Part model, mm, in its own coordinate system. Face numbers are marked on the shaded views. A direction names the side the tool comes from. Give positions to 0.01 mm unless a question says otherwise; leave off trailing zeros. Order: outer loops, then holes, each group sorted by start corner. A loop starts at its lowest first (then second) coordinate and runs counter-clockwise, first axis right, second up. Notation, with made-up numbers: (26.5, 45) -> (54.5, 45) arc R7 cw to (54.5, 51) -> close; hole circle Ø6 at (39, 77.25). An arc over 180 degrees is marked (long way). Write item = value, one per line. Start each with the question number.
Item 1: Flat gauge pins, fed straight in: P1, Ø3, axis at y = 25.5, z = -1, coming from the -X side; P2, Ø2, axis at y = -9.5, z = -5, coming from the -X side; P3, Ø7, axis at y = -23, z = -2.5, coming from the -X side; P4, Ø5, axis at y = -6, z = 5, coming from the -X side. Where does each tip first touch, or does it go through?
Item 2: Band-saw the part on B-B on x = 0. Write the cut outline in (y, z).
Item 3: Pull direction Z, two halves, no side cores. Call the marked faces 1, 2, 3 and 4: +Z half, -Z half, draft (parallel to the pull), parting line (faces both ways), or undercut.
Item 4: Drill centre lines: line 1 along Y through (x, z) = (0, 12.7); line 2 along Y through (x, z) = (0.5, 11.25); line 3 along X through (y, z) = (19, 10.5). Where is each one in solid material? Low to high.
Item 5: Band-saw the part on C-C on z = 3.5. Write the cut outline in (x, y), plus the area to 3 significant figures.
Item 6: Tool access for the marked faces 5, 6 and 7: list every direction of +Z, -Z, +X, -X, +Y, -Y with a clear straight run to the whole face (end or side of a thin tool).
Item 7: Band-saw the part on A-A on y = 0. Write the cut outline in (x, z), plus the area to 3 significant figures.
Item 8: Band-saw the part on D-D on y = -10. Write the cut outline in (x, z).
```python
from build123d import *

# Parameters (mm, degrees)
F3_W      = 25.4
F3_H      = 12.7
F4_DEPTH  = 72.39
F7_DEPTH  = 53.086
F10_DEPTH = 47.244


# Not quite as in the source:
# - a feature names something its author has since deleted; it is built from what else it names


with BuildPart() as f1:
    # F0 (on Front) → F1 (revolve)
    with BuildSketch(Plane.XZ):
        with BuildLine():
            ThreePointArc((23.01875, 10.7376509739), (25.4, 0), (23.01875, -10.7376509739))
            Line((23.01875, -10.7376509739), (23.01875, -14.2875))
            Line((23.01875, -14.2875), (26.611533725, -14.2875))
            ThreePointArc((26.611533725, -14.2875), (30.20441, 0), (26.611533725, 14.2875))
            Line((26.611533725, 14.2875), (23.01875, 14.2875))
            Line((23.01875, 14.2875), (23.01875, 10.7376509739))
        make_face()
    revolve(axis=Axis((0, 0, -4.5421977431), (0, 0, -1)))

    # F3 (on offset) → F4 (cut)
    with BuildSketch(Plane.XZ.offset(30.20441)):
        with BuildLine():
            ThreePointArc((12.7, 6.35), (0, 9.7529547439), (-12.7, 6.35))
            Line((-12.7, 6.35), (12.7, 6.35))
        make_face()
        Rectangle(F3_W, F3_H)
        with BuildLine():
            Line((12.7, -6.35), (-12.7, -6.35))
            ThreePointArc((-12.7, -6.35), (0, -9.7529547439), (12.7, -6.35))
        make_face()
    extrude(amount=-F4_DEPTH, mode=Mode.SUBTRACT)

    # F6 (on line) → F7 (cut, symmetric)
    with BuildSketch(Plane(origin=(0, 0, 0), x_dir=(0.5, -0.8660254038, 0), z_dir=(-0.8660254038, -0.5, 0))):
        with BuildLine():
            ThreePointArc((6.6390036837, -7.9375), (10.34796, 0), (6.6390036837, 7.9375))
            Line((6.6390036837, 7.9375), (-6.6390036837, 7.9375))
            ThreePointArc((-6.6390036837, 7.9375), (-10.34796, 0), (-6.6390036837, -7.9375))
            Line((-6.6390036837, -7.9375), (6.6390036837, -7.9375))
        make_face()
    extrude(amount=F7_DEPTH, both=True, mode=Mode.SUBTRACT)

    # F9 (on line) → F10 (cut, symmetric)
    with BuildSketch(Plane(origin=(0, 0, 0), x_dir=(-0.5, -0.8660254038, 0), z_dir=(-0.8660254038, 0.5, 0))):
        with BuildLine():
            ThreePointArc((6.6390036837, -7.9375), (10.34796, 0), (6.6390036837, 7.9375))
            Line((6.6390036837, 7.9375), (-6.6390036837, 7.9375))
            ThreePointArc((-6.6390036837, 7.9375), (-10.34796, 0), (-6.6390036837, -7.9375))
            Line((-6.6390036837, -7.9375), (6.6390036837, -7.9375))
        make_face()
    extrude(amount=F10_DEPTH, both=True, mode=Mode.SUBTRACT)


solid = f1.part
```
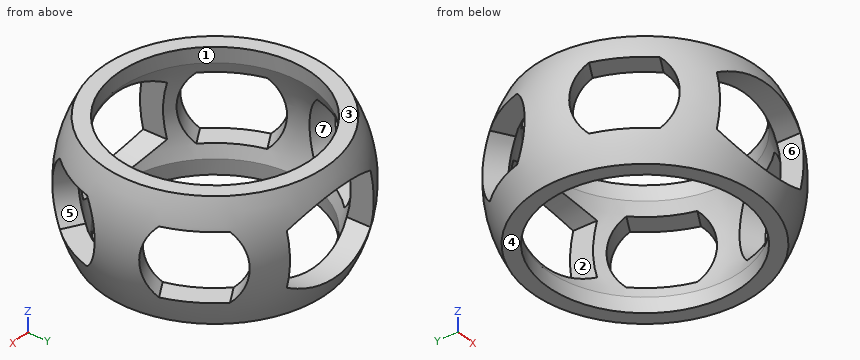
Values found:
q1.P1 = -18.31
q1.P2 = through
q1.P3 = -20.27
q1.P4 = -29.73
q2.outline = (-28.59, -9.75) arc R30.2 ccw to (-26.61, -14.29) -> (-23.02, -14.29) -> (-23.02, -10.74) arc R25.4 cw to (-23.45, -9.75) -> close; (-28.59, 9.75) -> (-23.45, 9.75) arc R25.4 cw to (-23.02, 10.74) -> (-23.02, 14.29) -> (-26.61, 14.29) arc R30.2 ccw to start; (23.02, -14.29) -> (26.61, -14.29) arc R30.2 ccw to (28.59, -9.75) -> (23.45, -9.75) arc R25.4 cw to (23.02, -10.74) -> close; (23.02, 10.74) arc R25.4 cw to (23.45, 9.75) -> (28.59, 9.75) arc R30.2 ccw to (26.61, 14.29) -> (23.02, 14.29) -> close
q3.face_1 = draft
q3.face_2 = undercut
q3.face_3 = +Z half
q3.face_4 = -Z half
q4.line_1 = -27.4 to -23.02, 23.02 to 27.4
q4.line_2 = -28.03 to -23.01, 23.01 to 28.03
q4.line_3 = -21 to -13.19, 13.19 to 21
q5.outline = (-29.44, -5.75) -> (-24.96, -3.16) arc R25.16 cw to (-24.96, 3.16) -> (-29.44, 5.75) arc R30 ccw to start; (-19.71, -22.62) arc R30 ccw to (-12.7, -27.18) -> (-12.7, -21.72) arc R25.16 cw to (-15.22, -20.03) -> close; (-19.71, 22.62) -> (-15.22, 20.03) arc R25.16 cw to (-12.7, 21.72) -> (-12.7, 27.18) arc R30 ccw to start; (12.7, -27.18) arc R30 ccw to (19.71, -22.62) -> (15.22, -20.03) arc R25.16 cw to (12.7, -21.72) -> close; (12.7, 21.72) arc R25.16 cw to (15.22, 20.03) -> (19.71, 22.62) arc R30 ccw to (12.7, 27.18) -> close; (24.96, -3.16) -> (29.44, -5.75) arc R30 ccw to (29.44, 5.75) -> (24.96, 3.16) arc R25.16 cw to start
q5.area = 198 mm^2
q6.face_5 = +X
q6.face_6 = +Y, -Y
q6.face_7 = +Y
q7.outline = (-26.61, -14.29) -> (-23.02, -14.29) -> (-23.02, -10.74) arc R25.4 cw to (-23.02, 10.74) -> (-23.02, 14.29) -> (-26.61, 14.29) arc R30.2 ccw to start; (23.02, -14.29) -> (26.61, -14.29) arc R30.2 ccw to (26.61, 14.29) -> (23.02, 14.29) -> (23.02, 10.74) arc R25.4 cw to (23.02, -10.74) -> close
q7.area = 275 mm^2
q8.outline = (-27.37, -7.94) arc R28.5 ccw to (-24.66, -14.29) -> (-20.73, -14.29) -> (-20.73, -10.74) arc R23.35 cw to (-21.96, -7.94) -> close; (-27.37, 7.94) -> (-21.96, 7.94) arc R23.35 cw to (-20.73, 10.74) -> (-20.73, 14.29) -> (-24.66, 14.29) arc R28.5 ccw to start; (20.73, -14.29) -> (24.66, -14.29) arc R28.5 ccw to (27.37, -7.94) -> (21.96, -7.94) arc R23.35 cw to (20.73, -10.74) -> close; (20.73, 10.74) arc R23.35 cw to (21.96, 7.94) -> (27.37, 7.94) arc R28.5 ccw to (24.66, 14.29) -> (20.73, 14.29) -> close
